Input: part model. Units: mm. Frame: model coordinates. Round coordinates to 2 decimals unless told otherwise and drop trailing zeros. Write each loop counter-clockwise with the first axis right and the second up, starting at its lowest first coordinate (ties: lowest second). Pieces come first, ordered by that corner, then holes. Notation, with made-up numbers: M 5.25,-12.5 L 12.25,-12.5 A11 ccw 12.25,8.5 Z; hole C 26,50.25 d9. An arc over 180 degrees is marked long. Write each question's results on one line, items separated by ' | '. Start each with the question number.
```python
from build123d import *

# Parameters (mm, degrees)
SKETCH1_W                 = 76
SKETCH1_H                 = 51
BOSS_EXTRUDE1_DEPTH       = 33
SKETCH2_R                 = 1.75
CUT_EXTRUDE1_DEPTH        = 57.420297766
SKETCH3_R                 = 0.5
IMU_CENTER_LOCATION_DEPTH = 5


with BuildPart() as part:
    # Sketch1 → Boss-Extrude1 (new body)
    with BuildSketch(Plane(origin=(0, 0, 0), x_dir=(1, 0, 0), z_dir=(0, 1, 0))):
        Rectangle(SKETCH1_W, SKETCH1_H)
    extrude(amount=BOSS_EXTRUDE1_DEPTH)

    # Sketch2 → Cut-Extrude1 (cut, through all)
    with BuildSketch(Plane(origin=(0, 0, 0), x_dir=(1, 0, 0), z_dir=(0, 1, 0))):
        with Locations(Location((-35, 22.15, 0), (0, 0, 270))):
            Circle(SKETCH2_R)
        with Locations(Location((35, 22.15, 0), (0, 0, 270))):
            Circle(SKETCH2_R)
        with Locations(Location((35, -22.15, 0), (0, 0, 270))):
            Circle(SKETCH2_R)
        with Locations(Location((-35, -22.15, 0), (0, 0, 270))):
            Circle(SKETCH2_R)
    extrude(amount=CUT_EXTRUDE1_DEPTH, mode=Mode.SUBTRACT)

    # Sketch3 → IMU_center_location (cut)
    with BuildSketch(Plane(origin=(0, 33, 0), x_dir=(1, 0, 0), z_dir=(0, 1, 0))):
        with Locations(Location((-4, -19.5, 0), (0, 0, 270))):
            Circle(SKETCH3_R)
    extrude(amount=-IMU_CENTER_LOCATION_DEPTH, mode=Mode.SUBTRACT)


solid = part.part
```
1. Cut plane B-B on z = 22.15. Output: boundary loops of the cut face in (x, y).
2. Draft query along Z for faces 1 (the face through (-1, 16, -25.5)), 2 (the face through (-38, 16, 0)), 3 (the face through (-34.92, 16.27, 20.4)). Return one class per face: +Z half, -Z half, draft (parallel to the pull), parting line (faces both ways), or undercut.
3. Contact query for flat-ended pins moving along their axis: P1, Ø5.5, axis at x = -35, z = -22.15, coming from the +Y side; P2, Ø2, axis at x = -35, z = 22.15, coming from the +Y side. Output: stop coordinate, or through.
4. Cut plane A-A on x = -35. Output: boundary loops of the cut face in (y, z).
5. Line query: L1, parallel to Z at x = 35, y = 21; L2, parallel to X at y = 21.5, z = 22.15; L3, parallel to X at y = 22.5, z = 21. Output: solid intervals per line, ascending. Write a range as from..to.
Answers follow:
1) outline: M -38,0 L -36.75,0 L -36.75,33 L -38,33 Z; M -33.25,0 L 33.25,0 L 33.25,33 L -33.25,33 Z; M 36.75,0 L 38,0 L 38,33 L 36.75,33 Z
2) face 1: -Z half | face 2: draft | face 3: undercut
3) P1: stops at y = 33 | P2: passes through
4) outline: M 0,-25.5 L 33,-25.5 L 33,-23.9 L 0,-23.9 Z; M 0,-20.4 L 33,-20.4 L 33,20.4 L 0,20.4 Z; M 0,23.9 L 33,23.9 L 33,25.5 L 0,25.5 Z
5) L1: z = -25.5..-23.9, -20.4..20.4, 23.9..25.5 | L2: x = -38..-36.75, -33.25..33.25, 36.75..38 | L3: x = -38..-36.32, -33.68..33.68, 36.32..38
